The model under review builds one solid part; all positions refer to its coordinate system, in mm. Face numbers are marked on the shaded views. A direction names the side the tool comes from. Round coordinates to 2 decimals unless told otherwise and drop trailing zeros. Order: outer loops, then holes, each group sorted by start corner. A loop starts at its lowest first (then second) coordinate and runs counter-clockwise, first axis right, second up. Notation, with made-up numbers: M 36.5,-6 L 53.5,-6 A36 cw 53.5,28 Z; hole C 82,-1.5 d7. An arc over 180 degrees is marked long. Answer as a JSON object with one key per item and string values. Group by question number.
1) Consider section B-B, the plane y = -19.5. Write out the cut boundary in (x, z) (1 decimal), then the cut area to 3 significant figures.
2) Consider section D-D, the plane x = -5. Write out the cut boundary in (y, z), then the cut area to 3 significant figures.
3) For the marked faces 1, 2 and 3, list the 3-axis set-ups (+Z, -Z, +X, -X, +Y, -Y) from which the entire face can be reached by the end or side of a thin tool; tool diameter is ignored.
4) Consider section A-A, the plane x = 0. Write out the cut boundary in (y, z).
5) To check wall thickness, follow line 1 (Z direction, x = -7, y = -19); line 2 (Y direction, x = 16, z = 6); line 3 (Y direction, x = -8.5, z = 12). State the ranges of each line that lie inside material, in increasing order.
6) Insertion check: pin 1 Ø1.6 at (x, z) = (-7.5, -13) entering from -Y; pin 2 Ø3.5 at (x, z) = (7, -13) entering from -Y; pin 3 Ø6 at (x, y) = (-13.5, -23.5) entering from +Z. Each pin has a flat end and moves straight along its axis. Give the tip position at first contact, or say it passes through.
```python
from build123d import *

# Parameters (mm, degrees)
SKETCH_R     = 18.5
PAD_DEPTH    = 24.5
SKETCH001_R  = 6
PAD001_DEPTH = 5
SKETCH002_R  = 3
PAD002_DEPTH = 15
SKETCH003_R  = 17.85
PAD003_DEPTH = 34
SKETCH004_W  = 1.450325
SKETCH004_H  = 4.868494
PAD004_DEPTH = 5.08
SKETCH005_R  = 1.5875
POCKET_DEPTH = 6.35


with BuildPart() as part:
    # Sketch → Pad (new body)
    with BuildSketch(Plane.XZ):
        Circle(SKETCH_R)
    extrude(amount=PAD_DEPTH)

    # Sketch001 (on Face3 of Pad) → Pad001 (join)
    with BuildSketch(Plane.XZ.offset(24.5)):
        Circle(SKETCH001_R)
    extrude(amount=PAD001_DEPTH)

    # Sketch002 (on Face5 of Pad001) → Pad002 (join)
    with BuildSketch(Plane.XZ.offset(29.5)):
        Circle(SKETCH002_R)
    extrude(amount=PAD002_DEPTH)

    # Sketch003 (on Face2 of Pad002) → Pad003 (join)
    with BuildSketch(Plane(origin=(0, 0, 0), x_dir=(1, 0, 0), z_dir=(0, 1, 0))):
        Circle(SKETCH003_R)
    extrude(amount=PAD003_DEPTH)

    # Sketch004 (on Face6 of Pad003) → Pad004 (join)
    with BuildSketch(Plane(origin=(0, 34, 0), x_dir=(1, 0, 0), z_dir=(0, 1, 0))):
        with Locations((-11.984146, 0)):
            Rectangle(SKETCH004_W, SKETCH004_H)
        with Locations((11.984146, 0)):
            Rectangle(SKETCH004_W, SKETCH004_H)
    extrude(amount=PAD004_DEPTH)

    # Sketch005 (on Face3 of Pad004) → Pocket (cut)
    with BuildSketch(Plane.XZ.offset(24.5)):
        with Locations((-7.49935, 12.989255)):
            Circle(SKETCH005_R)
        with Locations((-14.9987, 0)):
            Circle(SKETCH005_R)
        with Locations((-7.49935, -12.989255)):
            Circle(SKETCH005_R)
        with Locations((7.49935, -12.989255)):
            Circle(SKETCH005_R)
        with Locations((14.9987, 0)):
            Circle(SKETCH005_R)
        with Locations((7.49935, 12.989255)):
            Circle(SKETCH005_R)
    extrude(amount=-POCKET_DEPTH, mode=Mode.SUBTRACT)


solid = part.part
```
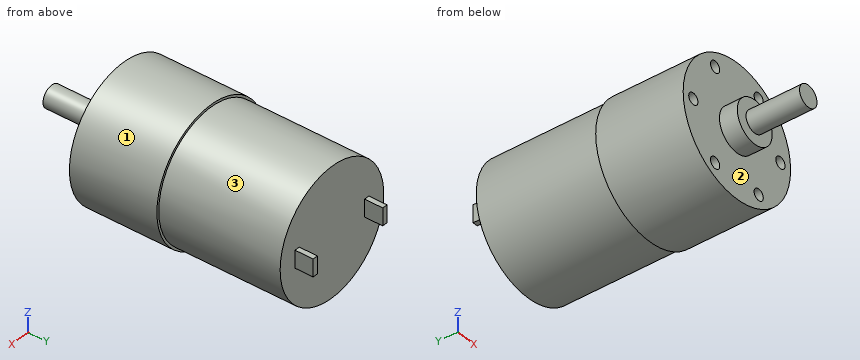
Results list:
{
 "1": {"outline": "C 0,0 d37; hole C -15,0 d3.2; hole C -7.5,-13 d3.2; hole C -7.5,13 d3.2; hole C 7.5,-13 d3.2; hole C 7.5,13 d3.2; hole C 15,0 d3.2", "area": "1,030 mm^2"},
 "2": {"outline": "M -29.5,-3.32 L -24.5,-3.32 L -24.5,-17.81 L 0,-17.81 L 0,-17.14 L 34,-17.14 L 34,17.14 L 0,17.14 L 0,17.81 L -24.5,17.81 L -24.5,3.32 L -29.5,3.32 Z", "area": "2,070 mm^2"},
 "3": {"face 1": "+Y, -Y", "face 2": "-Y", "face 3": "+Y"},
 "4": {"outline": "M -44.5,-3 L -29.5,-3 L -29.5,-6 L -24.5,-6 L -24.5,-18.5 L 0,-18.5 L 0,-17.85 L 34,-17.85 L 34,17.85 L 0,17.85 L 0,18.5 L -24.5,18.5 L -24.5,6 L -29.5,6 L -29.5,3 L -44.5,3 Z"},
 "5": {"line 1": "-17.12 to -14.5, -11.48 to 11.48, 14.5 to 17.12", "line 2": "-24.5 to 34", "line 3": "-18.15 to 34"},
 "6": {"pin 1": "y = -18.15", "pin 2": "y = -24.5", "pin 3": "z = 15.23"}
}
